```python
from build123d import *

# Parameters (mm, degrees)
SKETCH1_R                = 25
BOSS_EXTRUDE1_DEPTH      = 15
SKETCH1_3_R              = 12
BOSS_EXTRUDE2_DEPTH      = 40
BOSS_EXTRUDE4_REACH      = 105.385
BOSS_EXTRUDE4_END_RADIUS = 25
BOSS_EXTRUDE4_START      = 50
SKETCH4_W                = 40
SKETCH4_H                = 15
FILLET2_R                = 15
BOSS_EXTRUDE8_START      = 15
SKETCH7_R                = 4
BOSS_EXTRUDE8_DEPTH      = 15


with BuildPart() as part:
    # Sketch1 → Boss-Extrude1 (new body)
    with BuildSketch(Plane(origin=(0, 0, 0), x_dir=(1, 0, 0), z_dir=(0, 1, 0))):
        with Locations(Location((0, 0, 0), (0, 0, 270))):
            Circle(SKETCH1_R)
    extrude(amount=BOSS_EXTRUDE1_DEPTH)

    # Sketch1<3> → Boss-Extrude2 (add)
    with BuildSketch(Plane(origin=(0, 0, 0), x_dir=(1, 0, 0), z_dir=(0, 1, 0))):
        with Locations(Location((0, 0, 0), (0, 0, 270))):
            Circle(SKETCH1_3_R)
    extrude(amount=-BOSS_EXTRUDE2_DEPTH)

    # Boss-Extrude4: up to this cylinder (the profile starts outside it)
    boss_extrude4_end = Plane(origin=(0, 7.5, 0), z_dir=(0, -1, 0)) * Cylinder(BOSS_EXTRUDE4_END_RADIUS, 261.77, mode=Mode.PRIVATE)
    # Sketch4 → Boss-Extrude4 (add, up to the surface)
    with BuildSketch(Plane(origin=(0, 0, 0), x_dir=(0, 0, -1), z_dir=(1, 0, 0)).offset(BOSS_EXTRUDE4_START), mode=Mode.PRIVATE) as boss_extrude4_sk1:
        with Locations((0, 7.5)):
            Rectangle(SKETCH4_W, SKETCH4_H)
    boss_extrude4_tool1 = extrude(boss_extrude4_sk1.sketch, amount=-BOSS_EXTRUDE4_REACH, mode=Mode.PRIVATE) - boss_extrude4_end
    add(boss_extrude4_tool1.solids().sort_by_distance((50, 7.5, 0))[0])

    # Fillet2
    fillet2_edges = [part.edges().sort_by_distance(p)[0] for p in [
        (50, 7.5, -20),
        (50, 7.5, 20),
    ]]
    fillet(fillet2_edges, radius=FILLET2_R)

    # Sketch7 → Boss-Extrude8 (add)
    with BuildSketch(Plane(origin=(0, 0, 0), x_dir=(1, 0, 0), z_dir=(0, 1, 0)).offset(BOSS_EXTRUDE8_START)):
        with Locations(Location((20, 0, 0), (0, 0, 270))):
            Circle(SKETCH7_R)
    extrude(amount=BOSS_EXTRUDE8_DEPTH)


solid = part.part
```
Can you work these out from the model? Positions are in its coordinate system, mm. A direction names the side the tool comes from. Coordinates: 2 decimals unless noted, no trailing zeros. Loops run counter-clockwise (first coordinate to the right, second up) from the corner with the lowest first, then second, coordinate; pieces in that order, holes last. Notation, with made-up numbers: (86, 83) -> (105, 83) arc R21 ccw to (105, 109) -> close; hole circle Ø4 at (19, -22). An arc over 180 degrees is marked (long way). Put each result on its own line as item: value. Start each with the question number.
Q1. If I drill on line 1 (Y direction, x = -1, z = -18.5); line 2 (Y direction, x = 20, z = 1); line 3 (Z direction, x = 18.5, y = 10), over which ranges is the centre line in solid material (lowest first)? Write a range as [from, to].
Q2. I want a section at B-B (y = 14). Write out the boundary of the cut face in (x, z), plus the area to 3 significant figures.
Q3. I want a section at A-A (z = 0). Write out the boundary of the cut face in (x, y), plus the area to 4 significant figures.
Q4. I want a section at C-C (x = 0). Write out the boundary of the cut face in (y, z), plus the area to 3 significant figures.
Q5. I'm going to push flat-ended pins straight in: P1, Ø12, axis at x = 28, y = 7, coming from the +Z side; P2, Ø3, axis at y = -2, z = 3.5, coming from the +X side; P3, Ø3, axis at x = 3, y = -20.5, coming from the -Z side. Where does each tip first touch, or does it pass through?
Q6. I want a section at D-D (x = 20). Write out the boundary of the cut face in (y, z).
Q7. For faces 1 (the face through (3.604, -19.72, 11.446)), 2 (the face through (23.966, 22.395, -0.521)), 3 (the face through (25, 7, 20)), 4 (the face through (25, 7, -20)), which set-ups out of +Z, -Z, +X, -X, +Y, -Y let a thin tool reach every point of the face, with its end or its side?
Taken from the geometry:
1. line 1: y = [0, 15]
1. line 2: y = [0, 30]
1. line 3: z = [-20, 20]
2. outline: (15, -20) -> (35, -20) arc R15 ccw to (50, -5) -> (50, 5) arc R15 ccw to (35, 20) -> (15, 20) arc R25 ccw (long way) to start
2. area: 2,990 mm2
3. outline: (-25, 0) -> (-12, 0) -> (-12, -40) -> (12, -40) -> (12, 0) -> (50, 0) -> (50, 15) -> (24, 15) -> (24, 30) -> (16, 30) -> (16, 15) -> (-25, 15) -> close
3. area: 2,205 mm2
4. outline: (-40, -12) -> (0, -12) -> (0, -25) -> (15, -25) -> (15, 25) -> (0, 25) -> (0, 12) -> (-40, 12) -> close
4. area: 1,710 mm2
5. P1: stops at z = 20
5. P2: stops at x = 11.83
5. P3: stops at z = -11.91
6. outline: (0, -20) -> (15, -20) -> (15, -4) -> (30, -4) -> (30, 4) -> (15, 4) -> (15, 20) -> (0, 20) -> close
7. face 1: -Y
7. face 2: +Y
7. face 3: +Z, +X, +Y, -Y
7. face 4: -Z, +X, +Y, -Y
